from build123d import *

# Parameters (mm, degrees)
BOSS_EXTRUDE1_DEPTH      = 35
BOSS_EXTRUDE1_DEPTH_BACK = 35
HOLE1_D                  = 30
HOLE1_DEPTH              = 20


with BuildPart() as part:
    # Sketch1 → Boss-Extrude1 (new, two sides: drawn at the far end of the back side and taken through both)
    with BuildSketch(Plane.XY.offset(-BOSS_EXTRUDE1_DEPTH_BACK)):
        Polygon((-90, 0), (-90, 15), (-55, 15), (-55, 55), (55, 55), (55, 15), (90, 15), (90, 0), (40, 0), (40, 40), (-40, 40), (-40, 0), align=None)
    extrude(amount=BOSS_EXTRUDE1_DEPTH + BOSS_EXTRUDE1_DEPTH_BACK)

    # Sketch3 → Revolve1 (revolve)
    with BuildSketch(Plane.XY, mode=Mode.PRIVATE) as revolve1_sk:
        Polygon((0, 105), (35, 105), (19.713465927, 55), (0, 55), align=None)
    revolve(revolve1_sk.sketch.rotate(Axis((0, 0, 0), (0, 1, 0)), 90), axis=Axis((0, 0, 0), (0, 1, 0)))

    # Hole1
    with Locations(Plane(origin=(0, 105, 0), x_dir=(1, 0, 0), z_dir=(0, 1, 0))):
        with Locations((0, 0)):
            Hole(HOLE1_D / 2, depth=HOLE1_DEPTH)

    # Sketch7 → Hole2 (revolve, cut)
    with BuildSketch(Plane(origin=(0, 105, 0), x_dir=(0, 0, 1), z_dir=(1, 0, 0))):
        Polygon((0, 0), (0, 69.806884952), (8, 65), (8, 44.784609691), (20, 0), align=None)
    revolve(axis=Axis((0, 119.308894879, 0), (0, -1, 0)), mode=Mode.SUBTRACT)


solid = part.part
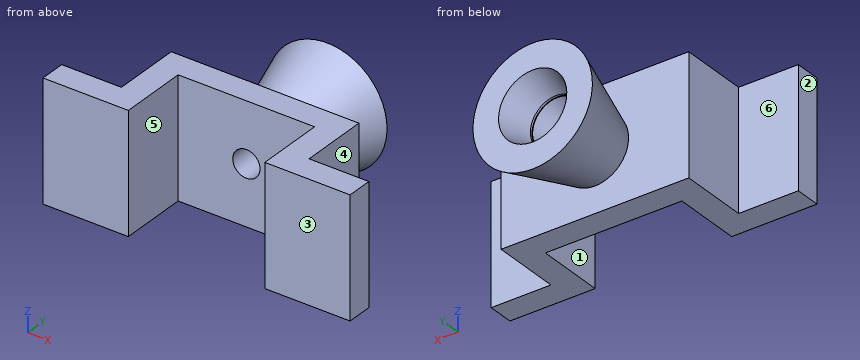
Verification items for the finished model (mm, model axes). Face numbers are marked on the shaded views. A direction names the side the tool comes from. Give positions to 0.01 mm unless a question says otherwise; leave off trailing zeros. Loops run counter-clockwise (first coordinate to the right, second up) from the corner with the lowest first, then second, coordinate; pieces in that order, holes last. Notation, with made-up numbers: (47, 47) - (86, 47) arc R9 ccw to (86, 62) - close; hole circle Ø9 at (27.5, 80.25). An arc over 180 degrees is marked (long way). Write each question's results on one line, items separated by ' | '.
1) Tool access check on the marked faces 4, 5 and 6. Record the directions out of +Z, -Z, +X, -X, +Y, -Y that give a thin tool (end or side, any length) a straight path to the whole face; none if there is none.
Solution:
face 4: +Z, -Z, +X, +Y | face 5: +Z, -Z, -Y | face 6: +Z, -Z, -X, +Y
2) Sectioned sample at C-C on z = 0. Record the boundary of the cut face in (x, y).
Solution:
outline: (-90, 0) - (-40, 0) - (-40, 40) - (-8, 40) - (-8, 60.22) - (-14.64, 85) - (-15, 85) - (-15, 86.34) - (-20, 105) - (-35, 105) - (-19.71, 55) - (-55, 55) - (-55, 15) - (-90, 15) - close; (8, 40) - (40, 40) - (40, 0) - (90, 0) - (90, 15) - (55, 15) - (55, 55) - (19.71, 55) - (35, 105) - (20, 105) - (15, 86.34) - (15, 85) - (14.64, 85) - (8, 60.22) - close
3) Material ranges on L1, parallel to X at y = 50, z = 0; L2, parallel to Y at x = -43, z = 8; L3, parallel to X at y = 6, z = -12.5, recorded low to high. Write a range as from..to.
Solution:
L1: -55..-8, 8..55 | L2: 0..55 | L3: -90..-40, 40..90
4) Depth check by flat-ended pin: P1, Ø3, axis at y = 15.5, z = 19, coming from the +X side; P2, Ø12, axis at y = 30, z = -10.5, coming from the +X side; P3, Ø21, axis at x = 0, z = 0, coming from the -Y side; P4, Ø5, axis at x = -53, z = -27, coming from the +Y side. Enter the tip coordinate at first touch or a pass-through.
Solution:
P1: x = 90 | P2: x = 55 | P3: y = 40 | P4: y = 55
5) Sectioned sample at A-A on y = 43. Record the boundary of the cut face in (x, z).
Solution:
outline: (-55, -35) - (55, -35) - (55, 35) - (-55, 35) - close; hole circle Ø16 at (0, 0)
6) Mould release check, pull along X, two halves, no side actions. Record for the marked faces 1, 2 and 3: pulls with the +X half, pulls with the -X half, needs draft (parallel to the pull), parting line crosses it, or undercut.
Solution:
face 1: undercut | face 2: pulls with the -X half | face 3: needs draft
7) Sectioned sample at D-D on x = -70. Record the boundary of the cut face in (y, z), plus the area to 3 significant figures.
Solution:
outline: (0, -35) - (15, -35) - (15, 35) - (0, 35) - close | area: 1,050 mm2
8) Sectioned sample at B-B on x = 0. Record the boundary of the cut face in (y, z), plus the area to 3 significant figures.
Solution:
outline: (40, -35) - (55, -35) - (55, -19.71) - (105, -35) - (105, -20) - (86.34, -15) - (85, -15) - (85, -14.64) - (60.22, -8) - (40, -8) - close; (40, 8) - (60.22, 8) - (85, 14.64) - (85, 15) - (86.34, 15) - (105, 20) - (105, 35) - (55, 19.71) - (55, 35) - (40, 35) - close | area: 2,210 mm2
